Source: three-view drawing plus pictorial views. Frame: mm from the lowest corner of the part. A direction names the side the tool comes from. Round coordinates to 2 decimals unless told otherwise and drop trailing zeros. Loops run counter-clockwise (first coordinate to the right, second up) from the corner with the lowest first, then second, coordinate; pieces in that order, holes last. Notation, with made-up numbers: M 69,29 L 74,29 A25 ccw 74,44 Z; hole C 88.25,11.25 d8. An arc over 180 degrees is marked long. Return JSON: item names as keys, results as strings. Group by question number.
1) Access query for the marked faces 1 and 2. Directions: +Z, -Z, +X, -X, +Y, -Y. A direction counts if a zero-diameter tool reaches every point of the face in a straight line with its end or side. Return the directions, or none.
2) Section B-B (y = 3). Output: boundary loops of the cut face in (x, z), plus the area to 3 significant figures.
3) Section C-C (z = 24.75). Output: boundary loops of the cut face in (x, y).
4) Section A-A (x = 39.5). Output: boundary loops of the cut face in (y, z).
5) Contact query for flat-ended pins moving along their axis: P1, Ø4, axis at x = 68, y = 8, coming from the +Z side; P2, Ø7, axis at y = 14, z = 41, coming from the -X side; P3, Ø1, axis at x = 35.5, z = 57, coming from the -Y side. Output: stop coordinate, or through.
6) Material intervals for line 1 (Y direction, x = 68.45, z = 49.75); line 2 (Z direction, x = 67.5, y = 12.75); line 3 (Z direction, x = 67.5, y = 19), sorted ascending. Write a range as from..to.
7) Section D-D (z = 37.5). Output: boundary loops of the cut face in (x, y).
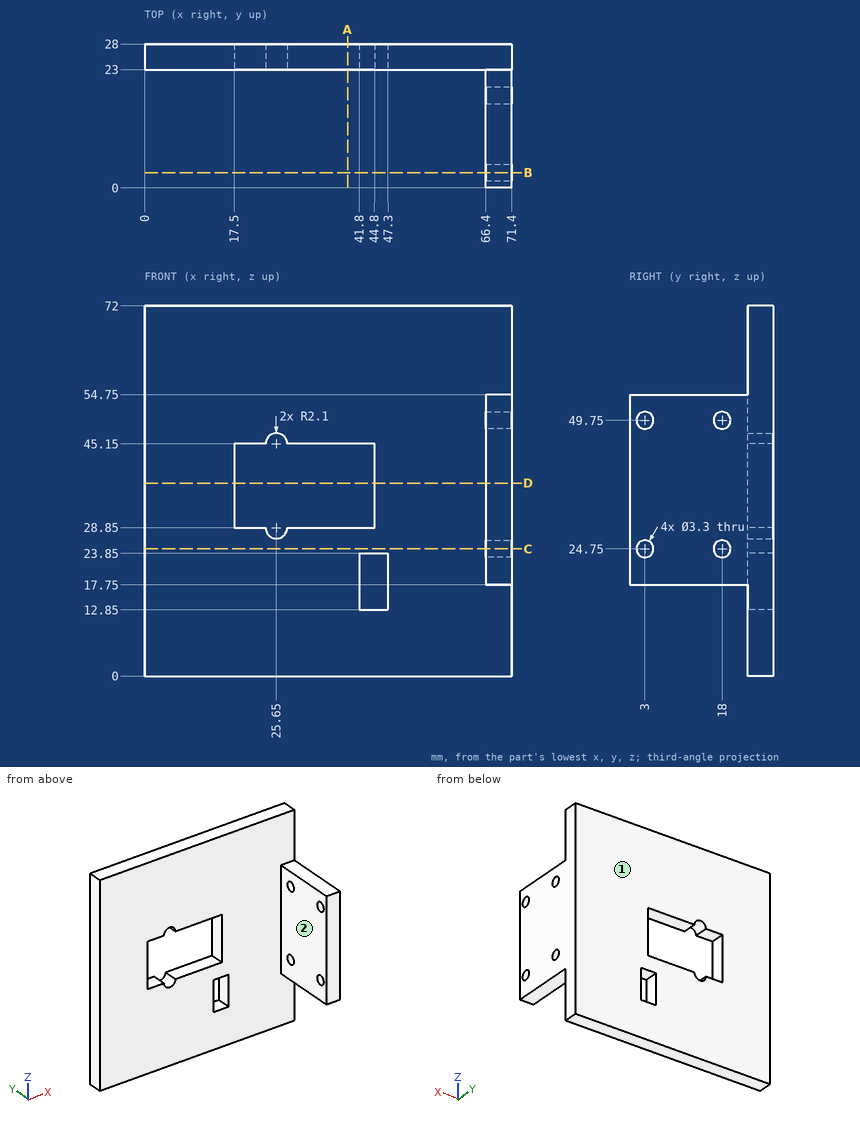
Returned:
{
 "1": {"face 1": "+Z, -Z, +X, -X, +Y", "face 2": "+Z, -Z, -X, -Y"},
 "2": {"outline": "M 66.4,17.75 L 71.4,17.75 L 71.4,23.1 L 66.4,23.1 Z; M 66.4,26.4 L 71.4,26.4 L 71.4,48.1 L 66.4,48.1 Z; M 66.4,51.4 L 71.4,51.4 L 71.4,54.75 L 66.4,54.75 Z", "area": "152 mm^2"},
 "3": {"outline": "M 0,23 L 66.4,23 L 66.4,19.65 L 71.4,19.65 L 71.4,28 L 0,28 Z; M 66.4,0 L 71.4,0 L 71.4,1.35 L 66.4,1.35 Z; M 66.4,4.65 L 71.4,4.65 L 71.4,16.35 L 66.4,16.35 Z"},
 "4": {"outline": "M 23,0 L 28,0 L 28,28.85 L 23,28.85 Z; M 23,45.15 L 28,45.15 L 28,72 L 23,72 Z"},
 "5": {"P1": "stops at z = 54.75", "P2": "stops at x = 66.4", "P3": "stops at y = 23"},
 "6": {"line 1": "y = 0..1.35, 4.65..16.35, 19.65..28", "line 2": "z = 17.75..54.75", "line 3": "z = 17.75..23.44, 26.06..48.44, 51.06..54.75"},
 "7": {"outline": "M 0,23 L 17.5,23 L 17.5,28 L 0,28 Z; M 44.8,23 L 66.4,23 L 66.4,0 L 71.4,0 L 71.4,28 L 44.8,28 Z"}
}
